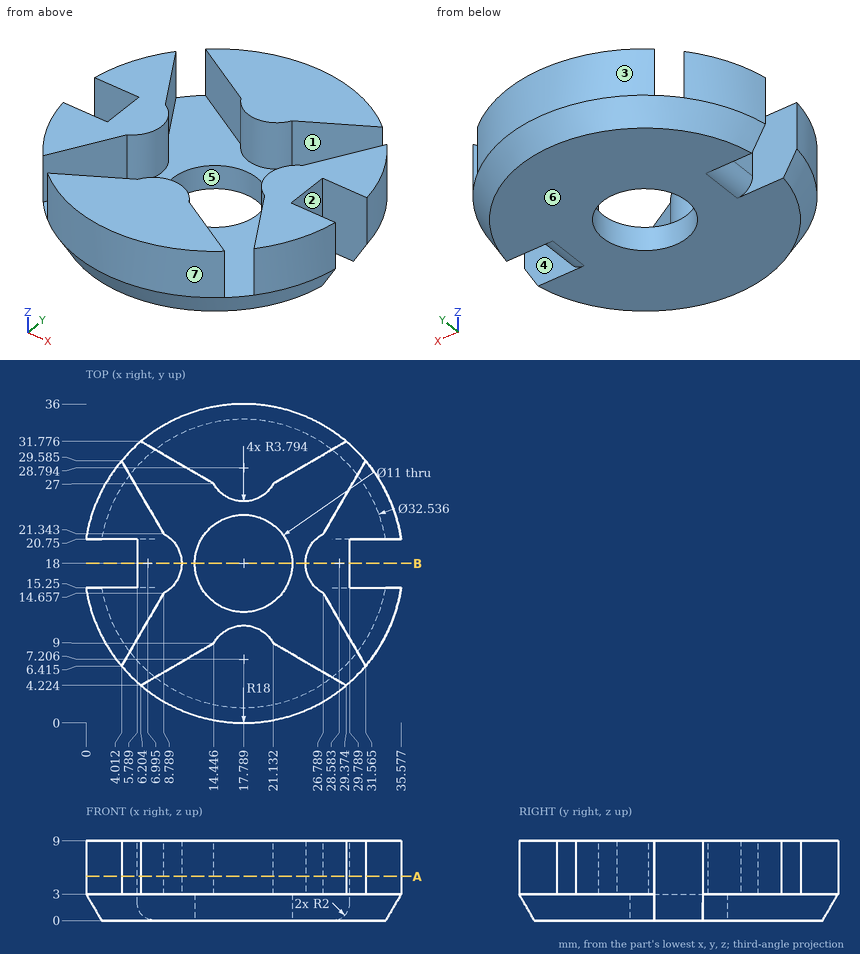
For this review, use the dimensioned drawing (mm, ordinates from the lowest corner) and the shaded views. A direction names the side the tool comes from. Coordinates: 2 decimals unless noted, no trailing zeros. Order: outer loops, then holes, each group sorted by start corner. A loop starts at its lowest first (then second) coordinate and runs counter-clockwise, first axis right, second up. Notation, with made-up numbers: M 39,19.5 L 74,19.5 A10 ccw 74,30.5 Z; hole C 85,35.5 d9. An arc over 180 degrees is marked long. Answer as a JSON object with one key per item and string values. Group by question number.
1) Add section A-A, the plane z = 5. Count the separate pieces of the cut face and the enclosed holes in it, then the cut area to 3 significant figures.
2) Add section B-B, the plane y = 18. Write out the cut boundary in (x, z).
3) Wall thickness on L1, parallel to Y at x = 10, z = 8.5 (1 decimal); L2, parallel to X at y = 26.5, z = 5 (1 decimal); L3, parallel to Z at x = 23, y = 20: over which ranges is each line inside the solid? List them lowest first.
4) Mouldability with a two-part tool opening along Y and no side actions: class the marked faces 4, 5, 6 and 7 as pulls with the +Y half, pulls with the -Y half, needs draft (parallel to the pull), parting line crosses it, or undercut.
5) Tool access review of the marked faces 1, 2 and 3: name each direction out of +Z, -Z, +X, -X, +Y, -Y from which nothing blocks a thin tool from reaching the whole face with its end or side.
6) For pin 1 (4 mm diameter, centred on x = 4.5, z = 5, fed in from +Y); pin 2 (4.5 mm diameter, centred on y = 18, z = 5.5, fed in from +X); pin 3 (1.5 mm diameter, centred on y = 3.5, z = 7.5, fed in from +X), all flat-tipped, find the tip position at first contact; note any pin that passes through.
Computed values:
{
 "1": {"separate pieces": "4", "enclosed holes": "0", "area": "526 mm^2"},
 "2": {"outline": "M 5.79,2 A2 ccw 7.79,0 L 12.29,0 L 12.29,3 L 10.79,3 L 10.79,9 L 5.79,9 Z; M 23.29,0 L 27.79,0 A2 ccw 29.79,2 L 29.79,9 L 24.79,9 L 24.79,3 L 23.29,3 Z"},
 "3": {"L1": "y = 1.8 to 6.4, 15.7 to 20.3, 29.6 to 34.2", "L2": "x = 1.9 to 5.8, 14.8 to 20.8, 29.8 to 33.7", "L3": "z = 0 to 3"},
 "4": {"face 4": "undercut", "face 5": "undercut", "face 6": "needs draft", "face 7": "pulls with the -Y half"},
 "5": {"face 1": "+Z", "face 2": "+Z, -Z, +X", "face 3": "+Z, -Z, +Y"},
 "6": {"pin 1": "stops at y = 32.02", "pin 2": "stops at x = 29.79", "pin 3": "stops at x = 29.37"}
}
